```python
from build123d import *

# Parameters (mm, degrees)
F0_W      = 133.35
F0_H      = 31.75
F1_DEPTH  = 31.75
F2_W      = 101.6
F2_H      = 25.4
F3_DEPTH  = 3.175
F5_DEPTH  = 3.175
F6_W      = 11.1125
F6_H      = 3.175
F7_DEPTH  = 3.175
F9_DEPTH  = 3.175
F11_DEPTH = 3.175
F14_DEPTH = 3.175
F15_DEPTH = 3.175
F17_DEPTH = 3.175
F19_DEPTH = 3.175
F21_DEPTH = 3.175
F22_W     = 95.25
F22_H     = 19.05
F23_DEPTH = 19.05


with BuildPart() as f1:
    # F0 (on Front) → F1 (new body)
    with BuildSketch(Plane.XZ):
        with Locations((66.675, 15.875)):
            Rectangle(F0_W, F0_H)
    extrude(amount=-F1_DEPTH)

    # F2 (on face) → F3 (cut)
    with BuildSketch(Plane.XZ):
        with Locations((53.975, 15.875)):
            Rectangle(F2_W, F2_H)
    extrude(amount=-F3_DEPTH, mode=Mode.SUBTRACT)

    # F4 (on face) → F5 (join)
    with BuildSketch(Plane.XZ.offset(-3.175)):
        Polygon((16.570325, 23.7998), (7.045325, 23.7998), (7.045325, 7.9375), (16.570325, 7.9375), (16.570325, 10.31875), (10.220325, 10.31875), (10.220325, 15.85595), (16.570325, 15.85595), (16.570325, 18.2372), (10.220325, 18.2372), (10.220325, 21.4122), (16.570325, 21.4122), align=None)
    extrude(amount=F5_DEPTH)

    # F6 (on face) → F7 (cut)
    with BuildSketch(Plane.XZ):
        with Locations((119.0625, 4.7625)):
            Rectangle(F6_W, F6_H)
    extrude(amount=-F7_DEPTH, mode=Mode.SUBTRACT)

    # F8 (on face) → F9 (cut)
    with BuildSketch(Plane.XZ):
        Polygon((124.61875, 28.212538), (113.50625, 28.212538), (113.50625, 23.450038), (116.68125, 23.450038), (116.68125, 25.037538), (121.972917, 25.037538), (116.68125, 9.525), (119.327083, 9.525), (124.61875, 25.037538), align=None)
    extrude(amount=-F9_DEPTH, mode=Mode.SUBTRACT)

    # F10 (on face) → F11 (join)
    with BuildSketch(Plane.XZ.offset(-3.175)):
        Polygon((23.61565, 23.7998), (20.44065, 23.7998), (20.44065, 7.9502), (29.96565, 7.9502), (29.96565, 11.1252), (23.61565, 11.1252), align=None)
    extrude(amount=F11_DEPTH)

    # F13 (on face) → F14 (join)
    with BuildSketch(Plane.XZ.offset(-3.175)):
        Polygon((43.360975, 23.7998), (33.835975, 23.7998), (33.835975, 7.9502), (43.360975, 7.9502), (43.360975, 10.3378), (37.010975, 10.3378), (37.010975, 15.8496), (43.360975, 15.8496), (43.360975, 18.2372), (37.010975, 18.2372), (37.010975, 21.4122), (43.360975, 21.4122), align=None)
    extrude(amount=F14_DEPTH)

    # F12 (on face) → F15 (join)
    with BuildSketch(Plane.XZ.offset(-3.175)):
        Polygon((50.504725, 23.7998), (46.535975, 23.7998), (46.535975, 7.9502), (49.710975, 7.9502), (49.710975, 18.146486), (51.69535, 7.9502), (54.87035, 7.9502), (56.854725, 18.146486), (56.854725, 7.9502), (60.029725, 7.9502), (60.029725, 23.7998), (56.060975, 23.7998), (53.28285, 9.525), align=None)
    extrude(amount=F15_DEPTH)

    # F16 (on face) → F17 (join)
    with BuildSketch(Plane.XZ.offset(-3.175)):
        Polygon((73.42505, 23.7998), (63.90005, 23.7998), (63.90005, 7.9502), (73.42505, 7.9502), (73.42505, 10.3378), (67.07505, 10.3378), (67.07505, 15.8496), (73.42505, 15.8496), (73.42505, 18.2372), (67.07505, 18.2372), (67.07505, 21.4122), (73.42505, 21.4122), align=None)
    extrude(amount=F17_DEPTH)

    # F18 (on face) → F19 (join)
    with BuildSketch(Plane.XZ.offset(-3.175)):
        Polygon((80.470375, 23.7998), (77.295375, 23.7998), (77.295375, 7.9502), (80.470375, 7.9502), (80.470375, 17.4752), (83.645375, 7.9502), (86.820375, 7.9502), (86.820375, 23.7998), (83.645375, 23.7998), (83.645375, 14.2748), align=None)
    extrude(amount=F19_DEPTH)

    # F20 (on face) → F21 (join)
    with BuildSketch(Plane.XZ.offset(-3.175)):
        Polygon((100.2157, 23.7998), (90.6907, 23.7998), (90.6907, 20.6248), (93.8657, 20.6248), (93.8657, 7.9502), (97.0407, 7.9502), (97.0407, 20.6248), (100.2157, 20.6248), align=None)
    extrude(amount=F21_DEPTH)

    # F22 (on face) → F23 (cut)
    with BuildSketch(Plane.XY.offset(31.75)):
        with Locations((66.675, 19.05)):
            Rectangle(F22_W, F22_H)
    extrude(amount=-F23_DEPTH, mode=Mode.SUBTRACT)


solid = f1.part
```
Check sheet for the modelled part. Datum: model origin and axes. Units: mm. A direction names the side the tool comes from. Give positions to 0.01 mm unless a question says otherwise; leave off trailing zeros. Order: outer loops, then holes, each group sorted by start corner. A loop starts at its lowest first (then second) coordinate and runs counter-clockwise, first axis right, second up. Notation, with made-up numbers: (-38, 4) -> (10, 4) arc R22 ccw to (10, 43) -> close; hole circle Ø2 at (-0.75, 54.25). An arc over 180 degrees is marked (long way). Use CSV: the item, a comma, the result in double quotes. Start each with the question number.
1) Set-up check for faces 1 (the face through (66, 28.575, 22)), 2 (the face through (85, 2, 7.95)): record each of +Z, -Z, +X, -X, +Y, -Y from which the full face is reachable in a straight line by a thin tool's end or side.
2) Sectioned sample at D-D, the plane x = 25.5. Record the boundary of the cut face in (y, z) (3 decimals).
3) Sectioned sample at C-C, the plane z = 5. Record the boundary of the cut face in (x, y) (3 decimals), plus the area to 3 significant figures.
4) Mould release check, pull along Z, two halves, no side actions. Record for faces 3 (the face through (95, 0, 18)), 4 (the face through (49.711, 2, 13)), 5 (the face through (66, 19, 12.7)): released by +Z, released by -Z, zero draft, split by the parting line, or undercut.
5) Sectioned sample at A-A, the plane z = 30.5. Record the boundary of the cut face in (x, y) (3 decimals), plus the area to 3 significant figures.
6) Sectioned sample at B-B, the plane y = 17.5. Record the boundary of the cut face in (x, z), plus the area to 3 significant figures.
7) Material ranges on line 1 (X direction, y = 12, z = 21); line 2 (Y direction, x = 99.5, z = 24) (3 decimals); line 3 (Z direction, x = 37, y = 19), recorded low to high. Write a range as from..to.
Recorded:
1,face 1,"+Z"
1,face 2,"-Y"
2,outline,"(0, 0) -> (31.75, 0) -> (31.75, 31.75) -> (28.575, 31.75) -> (28.575, 12.7) -> (9.525, 12.7) -> (9.525, 31.75) -> (0, 31.75) -> (0, 28.575) -> (3.175, 28.575) -> (3.175, 11.125) -> (0, 11.125) -> (0, 7.95) -> (3.175, 7.95) -> (3.175, 3.175) -> (0, 3.175) -> close"
3,outline,"(0, 0) -> (3.175, 0) -> (3.175, 3.175) -> (104.775, 3.175) -> (104.775, 0) -> (113.506, 0) -> (113.506, 3.175) -> (124.619, 3.175) -> (124.619, 0) -> (133.35, 0) -> (133.35, 31.75) -> (0, 31.75) -> close"
3,area,"3,880 mm2"
4,face 3,"zero draft"
4,face 4,"undercut"
4,face 5,"released by +Z"
5,outline,"(0, 0) -> (133.35, 0) -> (133.35, 31.75) -> (0, 31.75) -> close; hole (19.05, 9.525) -> (114.3, 9.525) -> (114.3, 28.575) -> (19.05, 28.575) -> close"
5,area,"2,420 mm2"
6,outline,"(0, 0) -> (133.35, 0) -> (133.35, 31.75) -> (114.3, 31.75) -> (114.3, 12.7) -> (19.05, 12.7) -> (19.05, 31.75) -> (0, 31.75) -> close"
6,area,"2,420 mm2"
7,line 1,"0..19.05, 114.3..133.35"
7,line 2,"3.175..9.525, 28.575..31.75"
7,line 3,"0..12.7"
